Could you check a few things on this model? Use its own coordinates, in mm. Round coordinates to 2 decimals unless told otherwise and drop trailing zeros. Write each loop counter-clockwise with the first axis right and the second up, starting at its lowest first coordinate (ties: lowest second). Pieces come first, ordered by that corner, then holes. Notation, with made-up numbers: (61, 45) - (72, 45) arc R22 ccw to (72, 55) - close; hole circle Ø11 at (16.25, 73). An arc over 180 degrees is marked (long way). Write each question's results on one line, items separated by ' | '. Start each with the question number.
(1) Imagine slicing it at B-B on x = 23. Write out the boundary of the cut face in (y, z), then the cut area to 3 significant figures.
(2) Please list where these lines run through material, in increasing order: line 1 (Y direction, x = 22.5, z = 3.75); line 2 (X direction, y = -8.5, z = 5); line 3 (X direction, y = -7.75, z = 3). Write a range as [from, to].
(3) Imagine slicing it at A-A on z = 3.25. Write out the boundary of the cut face in (x, y), then the cut area to 3 significant figures.
(4) For P1, Ø1.8, axis at x = 22.55, y = -7.7, coming from the +Z side, with a flat end and sliding along its axis, tell me the tip position at first contact or that it passes through.
(5) Imagine slicing it at C-C on y = 2.25. Write out the boundary of the cut face in (x, z), then the cut area to 3 significant figures.
Autodesk Inventor part; units mm, degrees
ref_plane "YZ Plane" through (0, 0, 0) normal (1, 0, 0) x (0, 1, 0)
ref_plane "XZ Plane" through (0, 0, 0) normal (0, 1, 0) x (-1, 0, 0)
ref_plane "XY Plane" through (0, 0, 0) normal (0, 0, 1) x (1, 0, 0)
sketch "Szkic1" plane through (0, 0, 0) normal (0, 0, 1) x (1, 0, 0)
  line L0 (-7.4523, 3.0496) -> (32.5477, 3.0496)
  line L1 (32.5477, 3.0496) -> (32.5477, -11.2004)
  line L2 (32.5477, -11.2004) -> (-7.4523, -11.2004)
  line L3 (-7.4523, -11.2004) -> (-7.4523, 3.0496)
  point P0 (0, 0)
  point P1 (2.5477, -7.7004)
  point P2 (22.5477, -7.7004)
  dimension "d0" = 40
  dimension "d1" = 14.25
  dimension "d2" = 3.5
  dimension "d3" = 3.5
  dimension "d4" = 10
  dimension "d5" = 10
extrude "Wyciągnięcie proste1" add sketch "Szkic1" along normal blind 8
hole "Otwór1" at (2.5477, -7.7004, 0) at (22.5477, -7.7004, 0) direction (0, 0, 1) diameter 3 end through all
chamfer "Faza1" distance 4 angle 45 2 edges at (-7.4523, -11.2004, 4) (32.5477, -11.2004, 4)
fillet "Zaokrąglenie1" radius 2 4 edges at (32.5477, -7.2004, 4) (28.5477, -11.2004, 4) (-3.4523, -11.2004, 4) (-7.4523, -7.2004, 4)
fillet "Zaokrąglenie4" radius 5 1 edges at (32.5477, 3.0496, 4)
fillet "Zaokrąglenie5" radius 2 1 edges at (-7.4523, 3.0496, 4)
properties part number "3DP_ABS_Y_Axis_Cable_Chain_Mounting_Bracket"
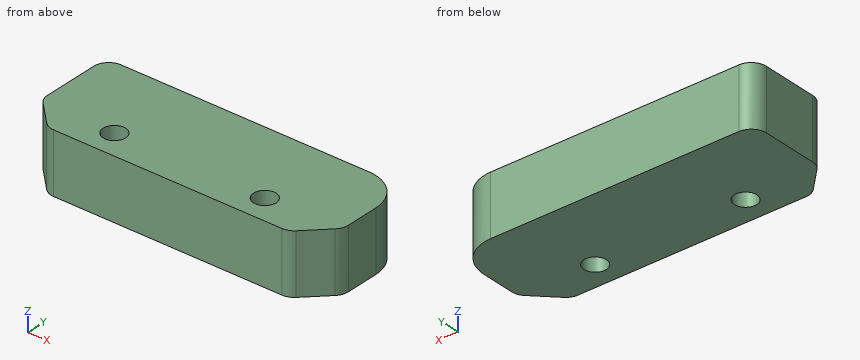
Response:
1) outline: (-11.2, 0) - (-9.13, 0) - (-9.13, 8) - (-11.2, 8) - close; (-6.27, 0) - (3.05, 0) - (3.05, 8) - (-6.27, 8) - close | area: 91.1 mm²
2) line 1: [-11.2, -9.2], [-6.2, 3.05] | line 2: [-6.15, 1.28], [3.82, 21.28], [23.82, 31.25] | line 3: [-6.9, 1.05], [4.05, 21.05], [24.05, 32]
3) outline: (-7.45, -6.37) arc R2 ccw to (-6.87, -7.79) - (-4.04, -10.61) arc R2 ccw to (-2.62, -11.2) - (27.72, -11.2) arc R2 ccw to (29.13, -10.61) - (31.96, -7.79) arc R2 ccw to (32.55, -6.37) - (32.55, -1.95) arc R5 ccw to (27.55, 3.05) - (-5.45, 3.05) arc R2 ccw to (-7.45, 1.05) - close; hole circle Ø3 at (2.55, -7.7); hole circle Ø3 at (22.55, -7.7) | area: 533 mm²
4) P1: through
5) outline: (-7.05, 0) - (30.26, 0) - (30.26, 8) - (-7.05, 8) - close | area: 298 mm²
